Model file for the job. Use its own axes, mm. A direction names the side the tool comes from. Round coordinates to 2 decimals unless told otherwise and drop trailing zeros. Write each loop counter-clockwise with the first axis right and the second up, starting at its lowest first coordinate (ties: lowest second). Pieces come first, ordered by that corner, then holes. Notation, with made-up numbers: (55.25, 6) - (114.25, 6) arc R30 cw to (114.25, 34) - close; hole circle Ø3 at (-33.5, 70). An arc over 180 degrees is marked (long way). Answer as a JSON object with one key per item and string values. Group by question number.
from build123d import *

# Parameters (mm, degrees)
SKETCH2_R           = 25.4
BOSS_EXTRUDE1_DEPTH = 15.875
SKETCH3_R           = 9.525
SKETCH3_R_2         = 4.7625
BOSS_EXTRUDE2_DEPTH = 9.525
SKETCH4_R           = 4.7625
CUT_EXTRUDE2_DEPTH  = 24.511
BOSS_EXTRUDE3_DEPTH = 3.175
FILLET1_R           = 2.54


with BuildPart() as part:
    # Sketch2 → Boss-Extrude1 (new body)
    with BuildSketch(Plane.XY):
        Circle(SKETCH2_R)
    extrude(amount=BOSS_EXTRUDE1_DEPTH)

    # Sketch3 → Boss-Extrude2 (add)
    with BuildSketch(Plane.XY.offset(15.875)):
        Circle(SKETCH3_R)
        Circle(SKETCH3_R_2, mode=Mode.SUBTRACT)
    extrude(amount=BOSS_EXTRUDE2_DEPTH)

    # Sketch4 → Cut-Extrude2 (cut)
    with BuildSketch(Plane.XY.offset(15.875)):
        Circle(SKETCH4_R)
    extrude(amount=-CUT_EXTRUDE2_DEPTH, mode=Mode.SUBTRACT)

    # Sketch5 → Boss-Extrude3 (add)
    with BuildSketch(Plane(origin=(0, 0, 0), x_dir=(-1, 0, 0), z_dir=(0, 0, -1))):
        Polygon((0, 4.7625), (1.27, 4.7625), (1.27, 0), (1.27, -4.7625), (0, -4.7625), (-1.27, -4.7625), (-1.27, 0), (-1.27, 4.7625), align=None)
    extrude(amount=-BOSS_EXTRUDE3_DEPTH)

    # Fillet1
    fillet1_edges = [part.edges().sort_by_distance(p)[0] for p in [
        (-9.525, 0, 15.875),
    ]]
    fillet(fillet1_edges, radius=FILLET1_R)


solid = part.part
(1) Slice it at D-D (y = -21). Write the cut outline in (x, z) (3 decimals).
(2) Slice it at C-C (z = 10.5). Write the cut outline in (x, y) (1 decimal).
(3) Drill centre lines: line 1 (Y direction, x = 0, z = 21.25) (1 decimal); line 2 (Y direction, x = 0, z = 6.25); line 3 (Z direction, x = 21.5, y = 1) (3 decimals). Where is each one in solid material? Low to high. Write a range as from..to.
(4) Pull direction X, two halves, no side cores. Call faces 4 (the flat face through (-1.27, 0, 2)), 5 (the cylindrical face through (-7.559, -5.796, 21.859)), 6 (the flat face through (0, 0, 3.175)), 7 (the flat face through (0, 0, 0)): pulls with the +X half, pulls with the -X half, needs draft (parallel to the pull), parting line crosses it, or undercut.
(5) Slice it at B-B (x = 0). Write the cut outline in (y, z) (1 decimal), then the cut area to 3 significant figures.
(6) Slice it at A-A (y = 0). Write the cut outline in (x, z) (1 decimal), then the cut area to 3 significant figures.
(7) Flat gauge pins, fed straight in: pin 1 (8 mm diameter, centred on x = 16.5, z = 17, fed in from -Y); pin 2 (12 mm diameter, centred on x = 9, z = 22, fed in from -Y); pin 3 (3 mm diameter, centred on x = -0.5, y = -1.5, fed in from +Z) (3 decimals). Where does each tip first touch, or does it go through?
(8) 3-axis set-ups, long thin cutter, end or side, ignore diameter. For faces 1 (the flat face through (1.27, 0, 2)), 2 (the flat face through (-4.4, 2.3, 25.4)), 3 (the flat face through (11, 6, 15.875)): which of +Z, -Z, +X, -X, +Y, -Y reach the whole face in a straight line?
Answer:
{
 "1": {"outline": "(-14.288, 0) - (14.288, 0) - (14.288, 15.875) - (-14.288, 15.875) - close"},
 "2": {"outline": "circle Ø50.8 at (0, 0); hole circle Ø9.5 at (0, 0)"},
 "3": {"line 1": "-9.5..-4.8, 4.8..9.5", "line 2": "-25.4..-4.76, 4.76..25.4", "line 3": "0..15.875"},
 "4": {"face 4": "undercut", "face 5": "parting line crosses it", "face 6": "undercut", "face 7": "needs draft"},
 "5": {"outline": "(-25.4, 0) - (25.4, 0) - (25.4, 15.9) - (12.1, 15.9) arc R2.5 cw to (9.5, 18.4) - (9.5, 25.4) - (4.8, 25.4) - (4.8, 3.2) - (-4.8, 3.2) - (-4.8, 25.4) - (-9.5, 25.4) - (-9.5, 18.4) arc R2.5 cw to (-12.1, 15.9) - (-25.4, 15.9) - close", "area": "779 mm²"},
 "6": {"outline": "(-25.4, 0) - (-4.8, 0) - (-4.8, 25.4) - (-9.5, 25.4) - (-9.5, 18.4) arc R2.5 cw to (-12.1, 15.9) - (-25.4, 15.9) - close; (-1.3, 0) - (1.3, 0) - (1.3, 3.2) - (-1.3, 3.2) - close; (4.8, 0) - (25.4, 0) - (25.4, 15.9) - (12.1, 15.9) arc R2.5 cw to (9.5, 18.4) - (9.5, 25.4) - (4.8, 25.4) - close", "area": "757 mm²"},
 "7": {"pin 1": "y = -22.02", "pin 2": "y = -9.04", "pin 3": "z = 3.175"},
 "8": {"face 1": "+Z, -Z", "face 2": "+Z, +X, -X, +Y, -Y", "face 3": "+Z"}
}
